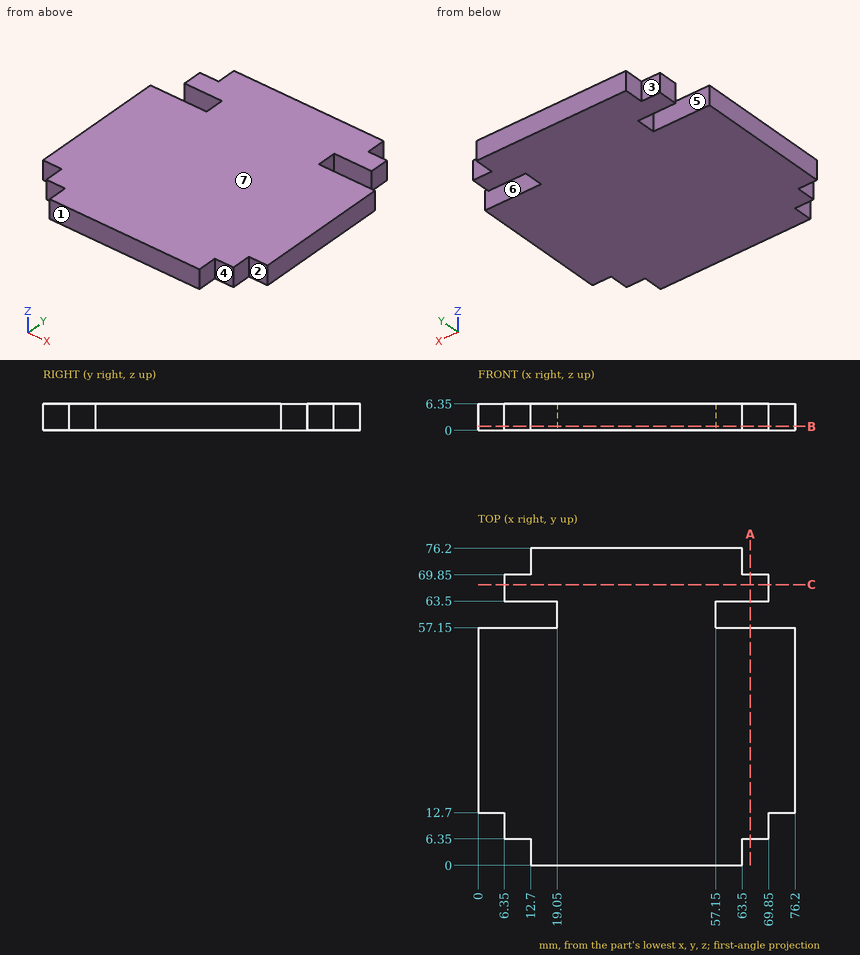
For this review, use the dimensioned drawing (mm, ordinates from the lowest corner) and the shaded views. A direction names the side the tool comes from. Give positions to 0.01 mm unless a question says otherwise; leave off trailing zeros. Write each loop counter-clockwise with the first axis right and the second up, starting at its lowest first coordinate (ties: lowest second). Pieces come first, ordered by that corner, then holes. Notation, with made-up numbers: M 19,40 L 70,40 A27 cw 70,66 Z; hole C 3,6.5 d1. An arc over 180 degrees is marked long. Write item = value, one per line. Start each with the question number.
Q1. Clearance check with flat-ended pins moving along their axes: pin 1 (3 mm diameter, centred on x = 68, z = 3, fed in from +Y); pin 2 (3 mm diameter, centred on y = 8.5, z = 2.5, fed in from +X); pin 3 (3 mm diameter, centred on y = 60, z = 4.5, fed in from +X). State where each tip first meets the part, or that it passes through.
Q2. For line 1 (Y direction, x = 69.5, z = 2.5); line 2 (Y direction, x = 58, z = 3.5); line 3 (X direction, y = 62.5, z = 4), list the stretches that pass through material, from the lowest coordinate up.
Q3. We need section C-C (y = 67.5). State the section outline as (x, z) points.
Q4. Mouldability with a two-part tool opening along Y and no side actions: class the marked faces 4, 5, 6 and 7 as released by +Y, released by -Y, zero draft, split by the parting line, or undercut.
Q5. We need section A-A (x = 65.5). State the section outline as (y, z) points, plus the area to 3 significant figures.
Q6. We need section B-B (z = 1). State the section outline as (x, y) points, plus the area to 3 significant figures.
Q7. Machinability: for the marked faces 1, 2 and 3, which of the approach directions +Z, -Z, +X, -X, +Y, -Y give a long, thin tool a straight path to every point of the face, cutting with its end or side? Answer none if there is none.
Result set:
q1.pin_1 = 69.85
q1.pin_2 = 69.85
q1.pin_3 = 57.15
q2.line_1 = 6.35 to 57.15, 63.5 to 69.85
q2.line_2 = 0 to 57.15, 63.5 to 76.2
q2.line_3 = 19.05 to 57.15
q3.outline = M 6.35,0 L 69.85,0 L 69.85,6.35 L 6.35,6.35 Z
q4.face_4 = released by -Y
q4.face_5 = undercut
q4.face_6 = undercut
q4.face_7 = zero draft
q5.outline = M 6.35,0 L 57.15,0 L 57.15,6.35 L 6.35,6.35 Z; M 63.5,0 L 69.85,0 L 69.85,6.35 L 63.5,6.35 Z
q5.area = 363 mm2
q6.outline = M 0,12.7 L 6.35,12.7 L 6.35,6.35 L 12.7,6.35 L 12.7,0 L 63.5,0 L 63.5,6.35 L 69.85,6.35 L 69.85,12.7 L 76.2,12.7 L 76.2,57.15 L 57.15,57.15 L 57.15,63.5 L 69.85,63.5 L 69.85,69.85 L 63.5,69.85 L 63.5,76.2 L 12.7,76.2 L 12.7,69.85 L 6.35,69.85 L 6.35,63.5 L 19.05,63.5 L 19.05,57.15 L 0,57.15 Z
q6.area = 5,080 mm2
q7.face_1 = +Z, -Z, +X, -X, -Y
q7.face_2 = +Z, -Z, +X, -Y
q7.face_3 = +Z, -Z, -X, +Y
